Build history of the part. All positions in model axes, mm. Face numbers are marked on the shaded views. A direction names the side the tool comes from. Coordinates: 2 decimals unless noted, no trailing zeros. Write each loop counter-clockwise with the first axis right and the second up, starting at its lowest first coordinate (ties: lowest second). Pieces come first, ordered by that corner, then holes. Notation, with made-up numbers: (27, 54) -> (66, 54) arc R17 cw to (66, 67) -> close; hole circle Ø6 at (-16.75, 42.5). An arc over 180 degrees is marked (long way). Write each question's results on one line, items separated by ' | '. Start each with the question number.
Q1. Tool access for the marked faces 1 and 2: list every direction of +Z, -Z, +X, -X, +Y, -Y with a clear straight run to the whole face (end or side of a thin tool).
Q2. Saw through at A-A on y = 0. Give the cut face in (x, z), and give its area (3 significant figures).
Q3. Saw through at B-B on x = 0. Give the cut face in (y, z), and give its area (3 significant figures).
Q4. Saw through at D-D on z = 1. Give the cut face in (x, y).
Q5. Drill centre lines: line 1 (Y direction, x = 0, z = 2.4); line 2 (Y direction, x = 0, z = 7.25); line 3 (Z direction, x = -6.25, y = 1). Where is each one in solid material? Low to high.
Q6. Saw through at C-C on z = 5. Give the cut face in (x, y).
Q7. Drop flat-ended pins along their axis: pin 1 Ø6 at (x, z) = (-8, 9) entering from +Y; pin 2 Ø8 at (x, z) = (5, 7) entering from +Y; pin 3 Ø6 at (x, y) = (0, 0) entering from -Z. Give the stop position or say it passes through.
from build123d import *

# Parameters (mm, degrees)
POCKET_DEPTH    = 12
SKETCH001_R     = 3.5
POCKET001_DEPTH = 4.5


with BuildPart() as part:
    # Sketch_knob → Revolution (revolve)
    with BuildSketch(Plane.XZ):
        with BuildLine():
            Line((0, 0), (0, 15.6))
            Line((0, 15.6), (11, 15.6))
            ThreePointArc((12, 14.6), (11.707107, 15.307107), (11, 15.6))
            Line((12, 14.6), (12, 6.6))
            ThreePointArc((11, 5.6), (11.707107, 5.892893), (12, 6.6))
            Line((11, 5.6), (5, 5.6))
            Line((5, 5.6), (5, 0))
            Line((5, 0), (0, 0))
        make_face()
    revolve(axis=Axis((0, 0, 0), (0, 0, 1)))

    # Sketch → Pocket (cut)
    with BuildSketch(Plane.XY):
        with BuildLine():
            ThreePointArc((-2.826659, 1.5), (0, -3.2), (2.826659, 1.5))
            Line((-2.826659, 1.5), (2.826659, 1.5))
        make_face()
    extrude(amount=POCKET_DEPTH, mode=Mode.SUBTRACT)

    # Sketch001 → Pocket001 (cut)
    with BuildSketch(Plane.XY):
        Circle(SKETCH001_R)
    extrude(amount=POCKET001_DEPTH, mode=Mode.SUBTRACT)


solid = part.part
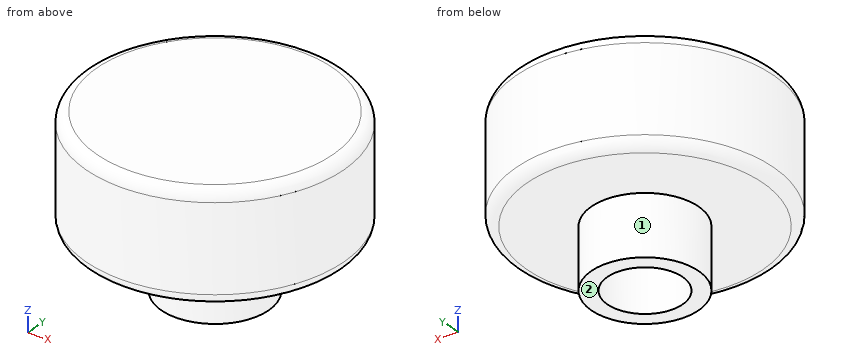
Returned:
1) face 1: -Z | face 2: -Z, +X, -X, +Y, -Y
2) outline: (-12, 6.6) arc R1 ccw to (-11, 5.6) -> (-5, 5.6) -> (-5, 0) -> (-3.5, 0) -> (-3.5, 4.5) -> (-3.2, 4.5) -> (-3.2, 12) -> (3.2, 12) -> (3.2, 4.5) -> (3.5, 4.5) -> (3.5, 0) -> (5, 0) -> (5, 5.6) -> (11, 5.6) arc R1 ccw to (12, 6.6) -> (12, 14.6) arc R1 ccw to (11, 15.6) -> (-11, 15.6) arc R1 ccw to (-12, 14.6) -> close | area: 216 mm2
3) outline: (-12, 6.6) arc R1 ccw to (-11, 5.6) -> (-5, 5.6) -> (-5, 0) -> (-3.5, 0) -> (-3.5, 4.5) -> (-3.2, 4.5) -> (-3.2, 12) -> (1.5, 12) -> (1.5, 4.5) -> (3.5, 4.5) -> (3.5, 0) -> (5, 0) -> (5, 5.6) -> (11, 5.6) arc R1 ccw to (12, 6.6) -> (12, 14.6) arc R1 ccw to (11, 15.6) -> (-11, 15.6) arc R1 ccw to (-12, 14.6) -> close | area: 228 mm2
4) outline: circle Ø10 at (0, 0); hole circle Ø7 at (0, 0)
5) line 1: y = -5 to -3.5, 3.5 to 5 | line 2: y = -12 to -3.2, 1.5 to 12 | line 3: z = 5.6 to 15.6
6) outline: circle Ø10 at (0, 0); hole (-2.83, 1.5) arc R3.2 ccw (long way) to (2.83, 1.5) -> close
7) pin 1: stops at y = 10.91 | pin 2: stops at y = 11.96 | pin 3: stops at z = 4.5
